```python
from build123d import *

# Parameters (mm, degrees)
F0_W     = 12
F0_H     = 40
F0_R     = 2.5
F0_R_2   = 12
F1_DEPTH = 12
F2_DEPTH = 11


with BuildPart() as f1:
    # F0 (on Top) → F1 (new body)
    with BuildSketch(Plane.XY):
        with Locations((14, 0)):
            Rectangle(F0_W, F0_H)
        with Locations((14, -12.73)):
            Circle(F0_R, mode=Mode.SUBTRACT)
        with Locations((14, 0)):
            Circle(F0_R, mode=Mode.SUBTRACT)
        with Locations((14, 12.73)):
            Circle(F0_R, mode=Mode.SUBTRACT)
        with BuildLine():
            Line((-9.206848, -16.694793), (8, -20))
            Line((8, -20), (8, 20))
            Line((8, 20), (-9.206848, 16.694793))
            ThreePointArc((-9.206848, 16.694793), (-23, 0), (-9.206848, -16.694793))
        make_face()
        with Locations((-6, 0)):
            Circle(F0_R_2, mode=Mode.SUBTRACT)
    extrude(amount=F1_DEPTH)

    # F0 (on Top) → F2 (join)
    with BuildSketch(Plane.XY):
        with Locations((-6, 0)):
            Circle(F0_R_2)
        with Locations((-6, 0)):
            Circle(F0_R, mode=Mode.SUBTRACT)
    extrude(amount=F2_DEPTH)


solid = f1.part
```
Work out the finished part from the listing and answer in its coordinate system (mm). A direction names the side the tool comes from. Give positions to 0.01 mm unless a question says otherwise; leave off trailing zeros. Order: outer loops, then holes, each group sorted by start corner. A loop starts at its lowest first (then second) coordinate and runs counter-clockwise, first axis right, second up.
1. Section B-B, the plane y = 0 is taken. Determine the outline of the cut face in (x, z).
Result sheet:
outline: (-23, 0) - (-8.5, 0) - (-8.5, 11) - (-18, 11) - (-18, 12) - (-23, 12) - close; (-3.5, 0) - (11.5, 0) - (11.5, 12) - (6, 12) - (6, 11) - (-3.5, 11) - close; (16.5, 0) - (20, 0) - (20, 12) - (16.5, 12) - close
2. Each of these flat-tipped pins is pushed along its axis until it touches: P1, Ø1.5, axis at y = 3.5, z = 1.5, coming from the -X side; P2, Ø1, axis at y = -6.5, z = 5, coming from the -X side. Where does it stop, or does it pass through?
Result sheet:
P1: stops at x = -22.78
P2: stops at x = -21.91
3. Section D-D, the plane x = -6 is taken. Determine the outline of the cut face in (y, z).
Result sheet:
outline: (-17.31, 0) - (-2.5, 0) - (-2.5, 11) - (-12, 11) - (-12, 12) - (-17.31, 12) - close; (2.5, 0) - (17.31, 0) - (17.31, 12) - (12, 12) - (12, 11) - (2.5, 11) - close
4. Section C-C, the plane z = 3.5 is taken. Determine the outline of the cut face in (x, y), and give its area (3 significant figures).
Result sheet:
outline: (-9.21, -16.69) - (8, -20) - (20, -20) - (20, 20) - (8, 20) - (-9.21, 16.69) arc R17 ccw to start; hole circle Ø5 at (-6, 0); hole circle Ø5 at (14, -12.73); hole circle Ø5 at (14, 0); hole circle Ø5 at (14, 12.73)
area: 1,380 mm2
5. For faces 5 (the flat face through (8, 0, 12)), 6 (the cylindrical face through (-15.523, -7.302, 11.493)), determine the directions among +Z, -Z, +X, -X, +Y, -Y from which every point of the face is accessible in a straight line to the end or side of a thin tool.
Result sheet:
face 5: +Z, +X, -X, +Y, -Y
face 6: +Z
6. Straight lines are drawn through the part: L1, parallel to Y at x = 13, z = 1.75; L2, parallel to X at y = 11, z = 11.75; L3, parallel to Z at x = 5, y = 3. For each, find the intervals that lie inside material, in ascending order.
Result sheet:
L1: y = -20 to -15.02, -10.44 to -2.29, 2.29 to 10.44, 15.02 to 20
L2: x = -18.96 to -10.8, -1.2 to 12.2, 15.8 to 20
L3: z = 0 to 11
7. Section A-A, the plane x = 14 is taken. Determine the outline of the cut face in (y, z), and give its area (3 significant figures).
Result sheet:
outline: (-20, 0) - (-15.23, 0) - (-15.23, 12) - (-20, 12) - close; (-10.23, 0) - (-2.5, 0) - (-2.5, 12) - (-10.23, 12) - close; (2.5, 0) - (10.23, 0) - (10.23, 12) - (2.5, 12) - close; (15.23, 0) - (20, 0) - (20, 12) - (15.23, 12) - close
area: 300 mm2
8. The mould has two halves that part along Y. Classify faces 1 (the cylindrical face through (11.5, 0.1, 5.9)), 2 (the cylindrical face through (-23, 0, 6)), 3 (the flat face through (-2, 0, 0)), 4 (the flat face through (14, -20, 6)): released by +Y, released by -Y, zero draft, split by the parting line, or undercut.
Result sheet:
face 1: undercut
face 2: split by the parting line
face 3: zero draft
face 4: released by -Y
